Model file for the job. Use its own axes, mm. A direction names the side the tool comes from. Coordinates: 2 decimals unless noted, no trailing zeros. Write each loop counter-clockwise with the first axis right and the second up, starting at its lowest first coordinate (ties: lowest second). Pieces come first, ordered by that corner, then holes.
Q1. Pull direction Y, two halves, no side cores. Call faces 3 (the cylindrical face through (-5.271, 6.463, 0.986)), 4 (the flat face through (-5, 15, -15)), 5 (the flat face through (-5, 4, 2)), 6 (the cylindrical face through (-0.6, 0.57, -14.79)): released by +Y, released by -Y, zero draft, split by the parting line, or undercut.
Q2. Which spindle directions (+Z, -Z, +X, -X, +Y, -Y) get a long thin tool onto all of the face, cutting with end or side? Do faces 1 (the flat face through (0, 7, -15)), 2 (the flat face through (-5, 7, 0)). Say none if no direction does.
Q3. Pin check, flat tip, straight feed: P1, Ø5, axis at y = 10, z = -4, coming from the +X side. Stop position of the tip, or through.
Q4. Drill centre lines: probe 1 along Z at (x, y) = (-7.75, 12.5); probe 2 along X at (y, z) = (1, -7); probe 3 along Y at (x, z) = (-1, -26.5). Where is each one in solid material? Low to high.
Q5. Band-saw the part on A-A, the plane z = -4.5. Write the cut outline in (x, y).
Q6. Band-saw the part on C-C, the plane y = 9.75. Write the cut outline in (x, z), plus the area to 3 significant figures.
Q7. Band-saw the part on D-D, the plane y = 7.5. Write the cut outline in (x, z).
Q8. Band-saw the part on B-B, the plane x = -5.75. Write the cut outline in (y, z).
Autodesk Inventor part; units mm, degrees
ref_plane "YZ Plane" through (0, 0, 0) normal (1, 0, 0) x (0, 1, 0)
ref_plane "XZ Plane" through (0, 0, 0) normal (0, 1, 0) x (-1, 0, 0)
ref_plane "XY Plane" through (0, 0, 0) normal (0, 0, 1) x (1, 0, 0)
sketch "Sketch1" plane through (0, 0, 0) normal (0, 1, 0) x (-1, 0, 0)
  point P0 (0, 0)
sketch "Sketch2" plane through (0, 0, 0) normal (0, 1, 0) x (-1, 0, 0)
  line L0 (0, 0) -> (10, 0)
  line L1 (10, 0) -> (10, -30)
  line L2 (10, -30) -> (0, -30)
  line L3 (0, -30) -> (0, 0)
  dimension "d0" = 10
  dimension "d1" = 30
extrude "Extrusion1" add sketch "Sketch2" along normal blind 15
fillet "Fillet1" radius 2 4 edges at (0, 15, -15) (-10, 15, -15) (0, 0, -15) (-10, 0, -15)
sketch "Sketch3" plane through (-8, 0, 0) normal (0, 0, 1) x (1, 0, 0)
  circle A0 centre (3.2708, 11.5209) radius 2.5
  circle A1 centre (3.2708, 4.0226) radius 2.5
  point P0 (8, 0)
  dimension "d5" = 5
  dimension "d6" = 5
extrude "Extrusion2" add sketch "Sketch3" along normal blind 2
properties part number "battery"
Answer sheet:
1. face 3: undercut
1. face 4: released by +Y
1. face 5: zero draft
1. face 6: released by -Y
2. face 1: +Z, -Z, +X, +Y, -Y
2. face 2: +Z
3. P1: stops at x = 0
4. probe 1: z = -30 to 0
4. probe 2: x = -9.73 to -0.27
4. probe 3: y = 0.27 to 14.73
5. outline: (-10, 2) arc R2 ccw to (-8, 0) - (-2, 0) arc R2 ccw to (0, 2) - (0, 13) arc R2 ccw to (-2, 15) - (-8, 15) arc R2 ccw to (-10, 13) - close
6. outline: (-10, -30) - (0, -30) - (0, 0) - (-2.96, 0) - (-2.96, 2) - (-6.49, 2) - (-6.49, 0) - (-10, 0) - close
6. area: 307 mm2
7. outline: (-10, -30) - (0, -30) - (0, 0) - (-10, 0) - close
8. outline: (0, -30) - (15, -30) - (15, 0) - (13.8, 0) - (13.8, 2) - (9.24, 2) - (9.24, 0) - (6.3, 0) - (6.3, 2) - (1.74, 2) - (1.74, 0) - (0, 0) - close
